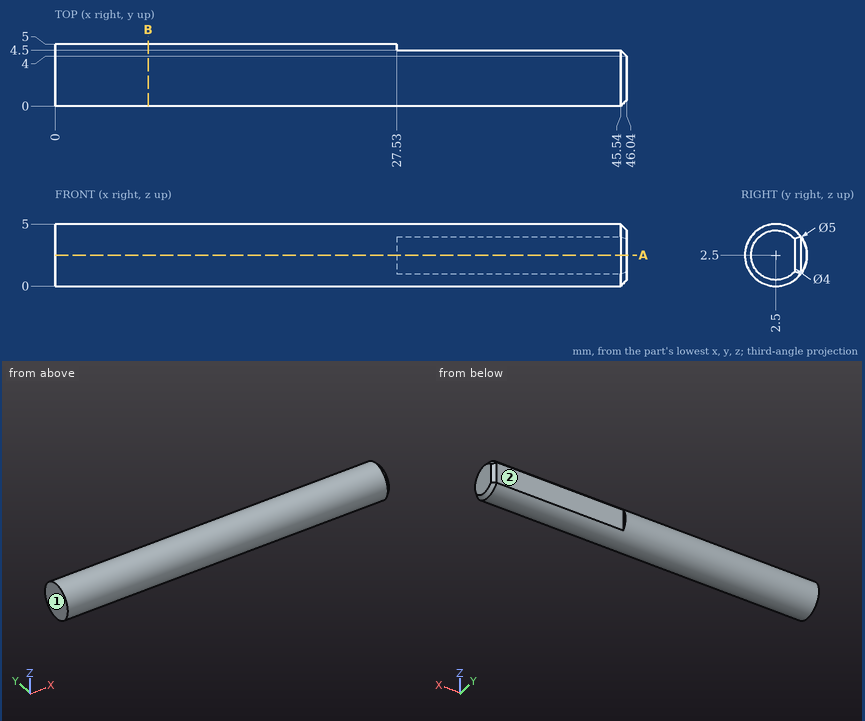
Can you work these out from the drawing? Everything is in mm from the part's minimum corner. A direction names the side the tool comes from. Give positions to 0.01 mm unless a question says otherwise; leave off trailing zeros. Order: outer loops, then holes, each group sorted by start corner. A loop starts at its lowest first (then second) coordinate and runs counter-clockwise, first axis right, second up. Notation, with made-up numbers: (5.5, 41.25) -> (27.5, 41.25) arc R17 ccw to (27.5, 59.25) -> close; hole circle Ø4 at (34.25, 26.25). An arc over 180 degrees is marked (long way). Return JSON: item names as keys, results as strings.
1. Imagine slicing it at A-A on z = 2.5. List the corners of the cut face in (x, y) for me.
Answer list:
{"outline": "(0, 0) -> (45.54, 0) -> (46.04, 0.5) -> (46.04, 4) -> (45.54, 4.5) -> (27.53, 4.5) -> (27.53, 5) -> (0, 5) -> close"}
2. Imagine slicing it at B-B on x = 7.5. List the corners of the cut face in (y, z) for me, then the cut area to 3 significant figures.
Answer list:
{"outline": "circle Ø5 at (2.5, 2.5)", "area": "19.6 mm2"}
3. I need wall thicknesses on line 1 (Y direction, x = 30.5, z = 2.7); line 2 (Y direction, x = 40, z = 0.8); line 3 (Z direction, x = 8.5, y = 4.65) (1 decimal). Which ranges of each line are inside material? Lowest first, please. Write a range as from..to.
Answer list:
{"line 1": "y = 0.01..4.5", "line 2": "y = 0.67..4.33", "line 3": "z = 1.2..3.8"}
4. For pin 1 Ø1.5 at (x, z) = (33, 2) entering from +Y; pin 2 Ø1 at (x, z) = (8, 4) entering from -Y; pin 3 Ø1.5 at (x, z) = (21.5, 3.5) entering from +Y, each with a flat end and sliding along its axis, tell me the tip position at first contact or that it passes through.
Answer list:
{"pin 1": "stops at y = 4.5", "pin 2": "stops at y = 0.21", "pin 3": "stops at y = 4.99"}
5. On a 3-axis mill with a long thin cutter (end or side, diameter ignored), from which of +Z, -Z, +X, -X, +Y, -Y can I reach the whole of each face in a straight line? I mean the marked faces 1 and 2. Say none if no direction works.
Answer list:
{"face 1": "+Z, -Z, -X, +Y, -Y", "face 2": "+Z, -Z, +X, +Y"}
